```python
from build123d import *

# Parameters (mm, degrees)
CROQUIS1_R              = 3.399999868
CROQUIS1_R_2            = 0.599999638
CROQUIS1_R_3            = 0.999999893
CROQUIS1_R_4            = 1.000000486
SALIENTE_EXTRUIR1_DEPTH = 3
CROQUIS2_W              = 16.5
CROQUIS2_H              = 2.5
SALIENTE_EXTRUIR2_DEPTH = 3
CORTAR_EXTRUIR1_DEPTH   = 3
CORTAR_EXTRUIR2_DEPTH   = 3
CROQUIS5_R              = 5
CROQUIS5_R_2            = 3.399999868
SALIENTE_EXTRUIR3_DEPTH = 3.5
REDONDEO1_R             = 3


with BuildPart() as part:
    # Croquis1 → Saliente-Extruir1 (new body)
    with BuildSketch(Plane(origin=(0, 0, 0), x_dir=(1, 0, 0), z_dir=(0, 1, 0))):
        with BuildLine():
            Line((36.746468572, 5.153075413), (36.746468572, 12.628075318))
            Line((36.746468572, 12.628075318), (-4.308066759, 12.628075318))
            ThreePointArc((-4.308066759, 12.628075318), (-35.260081681, 0.11801537), (-4.299942386, -12.371924682))
            Line((-4.299942386, -12.371924682), (36.746468572, -12.371924682))
            Line((36.746468572, -12.371924682), (36.746468572, -4.896924777))
            Line((36.746468572, -4.896924777), (26.846467047, -7.371924682))
            Line((26.846467047, -7.371924682), (26.846467047, 7.628075318))
            Line((26.846467047, 7.628075318), (36.746468572, 5.153075413))
        make_face()
        with Locations(Location((-17.253531302, 0.128075481, 0), (0, 0, 270))):
            Circle(CROQUIS1_R, mode=Mode.SUBTRACT)
        with Locations(Location((-17.253531676, 15.128075105, 0), (0, 0, 270))):
            Circle(CROQUIS1_R_2, mode=Mode.SUBTRACT)
        with Locations(Location((23.24646788, 6.128075095, 0), (0, 0, 270))):
            Circle(CROQUIS1_R_3, mode=Mode.SUBTRACT)
        with Locations(Location((23.246467992, -5.871925124, 0), (0, 0, 270))):
            Circle(CROQUIS1_R_4, mode=Mode.SUBTRACT)
        with Locations(Location((-6.646930036, 10.734677061, 0), (0, 0, 270))):
            Circle(CROQUIS1_R_2, mode=Mode.SUBTRACT)
        with Locations(Location((-2.25353164, 0.128075566, 0), (0, 0, 270))):
            Circle(CROQUIS1_R_2, mode=Mode.SUBTRACT)
        with Locations(Location((-6.646929684, -10.478526074, 0), (0, 0, 270))):
            Circle(CROQUIS1_R_2, mode=Mode.SUBTRACT)
        with Locations(Location((-17.253531179, -14.871924469, 0), (0, 0, 270))):
            Circle(CROQUIS1_R_2, mode=Mode.SUBTRACT)
        with Locations(Location((-27.860132819, -10.478526425, 0), (0, 0, 270))):
            Circle(CROQUIS1_R_2, mode=Mode.SUBTRACT)
        with Locations(Location((-32.253531215, 0.12807507, 0), (0, 0, 270))):
            Circle(CROQUIS1_R_2, mode=Mode.SUBTRACT)
        with Locations(Location((-27.860133171, 10.73467671, 0), (0, 0, 270))):
            Circle(CROQUIS1_R_2, mode=Mode.SUBTRACT)
    extrude(amount=SALIENTE_EXTRUIR1_DEPTH)

    # Croquis2 → Saliente-Extruir2 (add)
    with BuildSketch(Plane(origin=(0, 3, 0), x_dir=(1, 0, 0), z_dir=(0, 1, 0))):
        with BuildLine():
            Line((36.746468572, 12.628075318), (-4.308066759, 12.628075318))
            ThreePointArc((-4.308066759, 12.628075318), (-3.24436155, 11.423127984), (-2.292413315, 10.128075318))
            Line((-2.292413315, 10.128075318), (36.746468572, 10.128075318))
            Line((36.746468572, 10.128075318), (36.746468572, 12.628075318))
        make_face()
        with Locations((28.496468572, -11.121924682)):
            Rectangle(CROQUIS2_W, CROQUIS2_H)
    extrude(amount=SALIENTE_EXTRUIR2_DEPTH)

    # Croquis3 → Cortar-Extruir1 (cut)
    with BuildSketch(Plane.XY.offset(12.371924682)):
        Polygon((20.246468572, 3), (28.486468572, 6), (20.246468572, 6), align=None)
    extrude(amount=-CORTAR_EXTRUIR1_DEPTH, mode=Mode.SUBTRACT)

    # Croquis4 → Cortar-Extruir2 (cut)
    with BuildSketch(Plane(origin=(0, 0, -12.628075318), x_dir=(-1, 0, 0), z_dir=(0, 0, -1))):
        Polygon((4.308066759, 3), (4.308066759, 6), (-3.441933241, 6), align=None)
    extrude(amount=-CORTAR_EXTRUIR2_DEPTH, mode=Mode.SUBTRACT)

    # Croquis5 → Saliente-Extruir3 (add)
    with BuildSketch(Plane(origin=(0, 3, 0), x_dir=(1, 0, 0), z_dir=(0, 1, 0))):
        with Locations(Location((-17.253531302, 0.128075481, 0), (0, 0, 270))):
            Circle(CROQUIS5_R)
        with Locations(Location((-17.253531302, 0.128075481, 0), (0, 0, 270))):
            Circle(CROQUIS5_R_2, mode=Mode.SUBTRACT)
    extrude(amount=SALIENTE_EXTRUIR3_DEPTH)

    # Redondeo1
    redondeo1_edges = [part.edges().sort_by_distance(p)[0] for p in [
        (16.219200907, 0, -12.628075318),
        (16.223263093, 0, 12.371924682),
    ]]
    fillet(redondeo1_edges, radius=REDONDEO1_R - 0.0001)  # a hair under: the kernel refuses the full size


solid = part.part
```
Verification items for the finished model (mm, model axes). A direction names the side the tool comes from. Give positions to 0.01 mm unless a question says otherwise; leave off trailing zeros. Order: outer loops, then holes, each group sorted by start corner. A loop starts at its lowest first (then second) coordinate and runs counter-clockwise, first axis right, second up. Notation, with made-up numbers: (67.25, 23) -> (73.25, 23) arc R31 cw to (73.25, 62) -> close; hole circle Ø8 at (45, -8). An arc over 180 degrees is marked (long way). Use a Markdown table: item, result.
1) Section check A-A, the plane z = 2. Record the boundary of the cut face in (x, y).
Results:
| item | result |
|---|---|
| outline | (-35.13, 0) -> (-19.91, 0) -> (-19.91, 6.5) -> (-21.78, 6.5) -> (-21.78, 3) -> (-35.13, 3) -> close; (-14.6, 0) -> (26.85, 0) -> (26.85, 3) -> (-12.73, 3) -> (-12.73, 6.5) -> (-14.6, 6.5) -> close |
2) Section check B-B, the plane y = 4.75. Record the boundary of the cut face in (x, z).
Results:
| item | result |
|---|---|
| outline | circle Ø10 at (-17.25, -0.13); (0.21, -12.63) -> (36.75, -12.63) -> (36.75, -10.13) -> (0.21, -10.13) -> close; (25.05, 9.87) -> (36.75, 9.87) -> (36.75, 12.37) -> (25.05, 12.37) -> close; hole circle Ø6.8 at (-17.25, -0.13) |
3) Mould release check, pull along Z, two halves, no side actions. Record for faces 1 (the cylindrical face through (24.238, 1.479, 5.742)), 2 (the cylindrical face through (16.511, 0.855, 11.47)), 3 (the flat face through (31.866, 1.479, 6.117)), 4 (the flat face through (36.746, 2, 9)): pulls with the +Z half, pulls with the -Z half, needs draft (parallel to the pull), parting line crosses it, or undercut.
Results:
| item | result |
|---|---|
| face 1 | undercut |
| face 2 | pulls with the +Z half |
| face 3 | undercut |
| face 4 | needs draft |
4) Tool access check on faces 5 (the flat face through (26.846, 1, 0)), 6 (the flat face through (30, 4, 9.872)), 7 (the flat face through (0, 3, 0)), 8 (the cylindrical face through (15.93, 0.86, -11.73)), 9 (the flat face through (24.31, 4.48, 11.14)). Record the directions out of +Z, -Z, +X, -X, +Y, -Y that give a thin tool (end or side, any length) a straight path to the whole face; none if there is none.
Results:
| item | result |
|---|---|
| face 5 | +Y, -Y |
| face 6 | +X, -X, +Y |
| face 7 | +Y |
| face 8 | -Z, +X, -Y |
| face 9 | +Z, -X, +Y |
5) Section check D-D, the plane x = 29.5. Record the boundary of the cut face in (y, z), then the cut area to 3 significant figures.
Results:
| item | result |
|---|---|
| outline | (0, -9.63) arc R3 ccw to (3, -12.63) -> (6, -12.63) -> (6, -10.13) -> (3, -10.13) -> (3, -6.96) -> (0, -6.96) -> close; (0, 6.71) -> (3, 6.71) -> (3, 9.87) -> (6, 9.87) -> (6, 12.37) -> (3, 12.37) arc R3 ccw to (0, 9.37) -> close |
| area | 45.1 mm² |
6) Depth check by flat-ended pin: pin 1 Ø2 at (y, z) = (5.5, -4.5) entering from +X; pin 2 Ø0.9 at (x, y) = (9, 5) entering from -Z; pin 3 Ø1 at (x, y) = (28.5, 3.5) entering from +Z. Enter the tip coordinate at first touch or a pass-through.
Results:
| item | result |
|---|---|
| pin 1 | x = -13.56 |
| pin 2 | z = -12.63 |
| pin 3 | z = 12.37 |
7) Material ranges on probe 1 along Z at (x, y) = (33.5, 3.25); probe 2 along Y at (x, z) = (14.5, 9); probe 3 along X at (y, z) = (5.5, 2), recorded low to high.
Results:
| item | result |
|---|---|
| probe 1 | -12.63 to -10.13, 9.87 to 12.37 |
| probe 2 | 0 to 3 |
| probe 3 | -21.78 to -19.91, -14.6 to -12.73 |
